Input: part model. Units: mm. Frame: model coordinates. A direction names the side the tool comes from. Coordinates: 2 decimals unless noted, no trailing zeros. Loops run counter-clockwise (first coordinate to the right, second up) from the corner with the lowest first, then second, coordinate; pieces in that order, holes last.
(1) Contact query for flat-ended pins moving along their axis: P1, Ø1.5, axis at x = 152.5, y = 198.5, coming from the -Z side; P2, Ø1.5, axis at y = 199, z = 1.5, coming from the -X side; P3, Ø1.5, axis at x = 159.5, z = 0.5, coming from the +Y side; P4, Ø0.9, axis at x = 152.5, z = 1, coming from the -Y side. Output: stop coordinate, or through.
(2) Section B-B, the plane x = 148.5. Return loops of the section in (y, z), then the cut area to 3 significant figures.
(3) Set-up query: faces 1 (the face through (161.49, 210.54, 1.48)), 2 (the face through (152, 202.824, 1)), 3 (the face through (156.717, 198, 1)). Return all of +Z, -Z, +X, -X, +Y, -Y with unobstructed straight access to the full face (end or side cutting, diameter ignored); none if empty.
(4) Section C-C, the plane y = 197. Return loops of the section in (x, z), then the cut area to 3 significant figures.
(5) Mould query, pull axis Y, two halves, no side actions, for faces 4 (the face through (147.844, 207.39, 1.479)), 5 (the face through (153.842, 201, 1)), 6 (the face through (156.844, 207.39, 1.479)), 7 (the face through (144.843, 207.225, 1.479)). Classes: released by +Y, released by -Y, zero draft, split by the parting line, or undercut.
(6) Section A-A, the plane z = 1.05. Return loops of the section in (x, y).
(7) Section D-D, the plane y = 206.5. Return loops of the section in (x, z).
(8) Line query: L1, parallel to Y at x = 158.25, z = 1.95; L2, parallel to Y at x = 159.5, z = 2.25; L3, parallel to Y at x = 152.75, z = 0.95. Output: solid intervals per line, ascending.
```python
from build123d import *

# Parameters (mm, degrees)
MODEL_R                 = 1.5
SALIENTE_EXTRUIR1_DEPTH = 3


with BuildPart() as part:
    # Model → Saliente-Extruir1 (new body)
    with BuildSketch(Plane.XY):
        with BuildLine():
            Line((149.34213351, 211.823953209), (158.34213351, 211.823953209))
            ThreePointArc((158.34213351, 211.823953209), (161.524114025, 210.505933724), (162.84213351, 207.323953209))
            Line((162.84213351, 207.323953209), (162.84213351, 198.323953209))
            ThreePointArc((162.84213351, 198.323953209), (158.34213351, 193.823953209), (153.84213351, 198.323953209))
            Line((153.84213351, 198.323953209), (153.84213351, 202.823953209))
            Line((153.84213351, 202.823953209), (149.34213351, 202.823953209))
            ThreePointArc((149.34213351, 202.823953209), (144.84213351, 207.323953209), (149.34213351, 211.823953209))
        make_face()
        with Locations((149.34213351, 207.323953209)):
            Circle(MODEL_R, mode=Mode.SUBTRACT)
        with Locations((158.34213351, 207.323953209)):
            Circle(MODEL_R, mode=Mode.SUBTRACT)
        with BuildLine():
            Line((156.71713351, 195.823953209), (156.71713351, 200.823953209))
            ThreePointArc((156.71713351, 200.823953209), (156.936803424, 201.354283295), (157.46713351, 201.573953209))
            Line((157.46713351, 201.573953209), (159.21713351, 201.573953209))
            ThreePointArc((159.21713351, 201.573953209), (159.747463595, 201.354283295), (159.96713351, 200.823953209))
            Line((159.96713351, 200.823953209), (159.96713351, 195.823953209))
            ThreePointArc((159.96713351, 195.823953209), (159.747463595, 195.293623123), (159.21713351, 195.073953209))
            Line((159.21713351, 195.073953209), (157.46713351, 195.073953209))
            ThreePointArc((157.46713351, 195.073953209), (156.936803424, 195.293623123), (156.71713351, 195.823953209))
        make_face(mode=Mode.SUBTRACT)
    extrude(amount=SALIENTE_EXTRUIR1_DEPTH)


solid = part.part
```
Report:
1. P1: passes through
1. P2: stops at x = 153.84
1. P3: stops at y = 211.81
1. P4: stops at y = 202.82
2. outline: (202.9, 0) - (206.08, 0) - (206.08, 3) - (202.9, 3) - close; (208.57, 0) - (211.74, 0) - (211.74, 3) - (208.57, 3) - close
2. area: 19.1 mm2
3. face 1: +Z, -Z, +X, +Y
3. face 2: +Z, -Z, -X, -Y
3. face 3: +Z, -Z
4. outline: (154.04, 0) - (156.72, 0) - (156.72, 3) - (154.04, 3) - close; (159.97, 0) - (162.64, 0) - (162.64, 3) - (159.97, 3) - close
4. area: 16.1 mm2
5. face 4: undercut
5. face 5: zero draft
5. face 6: undercut
5. face 7: split by the parting line
6. outline: (149.34, 202.82) - (153.84, 202.82) - (153.84, 198.32) arc R4.5 ccw to (162.84, 198.32) - (162.84, 207.32) arc R4.5 ccw to (158.34, 211.82) - (149.34, 211.82) arc R4.5 ccw to start; hole circle Ø3 at (149.34, 207.32); hole (156.72, 195.82) arc R0.75 ccw to (157.47, 195.07) - (159.22, 195.07) arc R0.75 ccw to (159.97, 195.82) - (159.97, 200.82) arc R0.75 ccw to (159.22, 201.57) - (157.47, 201.57) arc R0.75 ccw to (156.72, 200.82) - close; hole circle Ø3 at (158.34, 207.32)
7. outline: (144.92, 0) - (148.09, 0) - (148.09, 3) - (144.92, 3) - close; (150.6, 0) - (157.09, 0) - (157.09, 3) - (150.6, 3) - close; (159.6, 0) - (162.84, 0) - (162.84, 3) - (159.6, 3) - close
8. L1: y = 193.82 to 195.07, 201.57 to 205.83, 208.82 to 211.82
8. L2: y = 193.98 to 195.13, 201.52 to 206.37, 208.28 to 211.67
8. L3: y = 202.82 to 211.82
